from build123d import *

# Parameters (mm, degrees)
SKETCH1_R           = 3.175
BOSS_EXTRUDE1_DEPTH = 1.5875
FILLET1_R           = 3.175
FILLET2_R           = 1.5875


with BuildPart() as part:
    # Sketch1 → Boss-Extrude1 (new body)
    with BuildSketch(Plane(origin=(0, 0, 0), x_dir=(1, 0, 0), z_dir=(0, 1, 0))):
        with BuildLine():
            Line((-30.943444248, 0), (12.7, 0))
            Line((12.7, 0), (12.7, 1.5875))
            Line((12.7, 1.5875), (38.1, 1.5875))
            Line((38.1, 1.5875), (38.1, 61.9125))
            Line((38.1, 61.9125), (28.575, 61.9125))
            Line((28.575, 61.9125), (28.575, 11.1125))
            Line((28.575, 11.1125), (12.7, 11.1125))
            Line((12.7, 11.1125), (12.7, 12.7))
            Line((12.7, 12.7), (-30.943444248, 12.7))
            ThreePointArc((-30.943444248, 12.7), (-31.75, 6.35), (-30.943444248, 0))
        make_face()
        with Locations(Location((-6.35, 6.35, 0), (0, 0, 270))):
            Circle(SKETCH1_R, mode=Mode.SUBTRACT)
    extrude(amount=BOSS_EXTRUDE1_DEPTH)

    # Fillet1
    fillet1_edges = [part.edges().sort_by_distance(p)[0] for p in [
        (28.575, 0.79375, -11.1125),
        (28.575, 0.79375, -61.9125),
        (38.1, 0.79375, -61.9125),
        (38.1, 0.79375, -1.5875),
    ]]
    fillet(fillet1_edges, radius=FILLET1_R)

    # Fillet2
    fillet2_edges = [part.edges().sort_by_distance(p)[0] for p in [
        (12.7, 0.79375, 0),
        (12.7, 0.79375, -12.7),
    ]]
    fillet(fillet2_edges, radius=FILLET2_R - 0.0001)  # a hair under: the kernel refuses the full size


solid = part.part
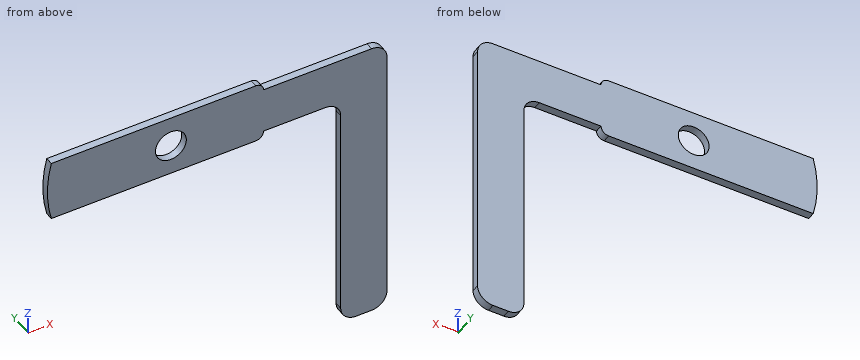
Model file for the job. Use its own axes, mm. Round coordinates to 2 decimals unless told otherwise and drop trailing zeros. Loops run counter-clockwise (first coordinate to the right, second up) from the corner with the lowest first, then second, coordinate; pieces in that order, holes last. Notation, with made-up numbers: (18, -33.5) - (25, -33.5) arc R9 cw to (25, -26.5) - close; hole circle Ø1 at (-13.5, 14.5). An arc over 180 degrees is marked (long way). Write each question's results on one line, items separated by ' | '.
(1) Wall check: L1, parallel to X at y = 1.05, z = -6.35 (3 decimals); L2, parallel to X at y = 0.2, z = -41 (3 decimals); L3, parallel to Z at x = 25.5, y = 0.25. Give the ranges that are in metal, low to high.
Answer below:
L1: x = -31.75 to -9.525, -3.175 to 38.1 | L2: x = 28.575 to 38.1 | L3: z = -11.11 to -1.59
(2) Saw through at B-B, the plane x = -6.35. List the corners of the cut face in (y, z) (1 decimal).
Answer below:
outline: (0, -12.7) - (1.6, -12.7) - (1.6, -9.5) - (0, -9.5) - close; (0, -3.2) - (1.6, -3.2) - (1.6, 0) - (0, 0) - close
(3) Pin check, flat tips, straight feed: pin 1 (0.5 mm diameter, centred on x = 18.5, y = 1, fed in from -Z); pin 2 (0.8 mm diameter, centred on y = 0.5, z = -39.5, fed in from -X) (3 decimals); pin 3 (0.5 mm diameter, centred on x = 23, y = 0.5, fed in from +Z); pin 4 (4 mm diameter, centred on x = -6.35, z = -6.35, fed in from -Y). Stop position of each tip, or through.
Answer below:
pin 1: stops at z = -11.11 | pin 2: stops at x = 28.575 | pin 3: stops at z = -1.59 | pin 4: passes through
(4) Saw through at D-D, the plane x = -22.5. List the corners of the cut face in (y, z), then the cut area to 3 significant figures.
Answer below:
outline: (0, -12.7) - (1.59, -12.7) - (1.59, 0) - (0, 0) - close | area: 20.2 mm^2
